CAD build for the part. Positions are in the model's coordinates, mm. A direction names the side the tool comes from. Coordinates: 2 decimals unless noted, no trailing zeros. Order: outer loops, then holes, each group sorted by start corner. A loop starts at its lowest first (then second) coordinate and runs counter-clockwise, first axis right, second up. Notation, with made-up numbers: (56.5, 69.25) - (77.5, 69.25) arc R32 cw to (77.5, 104.25) - close; hole circle Ø10 at (85, -22.75). An arc over 180 degrees is marked (long way). Use one line per item in the form item = value.
```python
from build123d import *

# Parameters (mm, degrees)
SKETCH_R           = 56.5
PAD_DEPTH          = 35
SKETCH001_R        = 55
POCKET_DEPTH       = 33
SKETCH002_R        = 6.9
PAD001_DEPTH       = 110
CHAMFER_SIZE       = 1
CHAMFER001_SIZE    = 1
SKETCH006_R        = 10
POCKET002_DEPTH    = 5
POLARPATTERN_COUNT = 6


with BuildPart() as part:
    # Sketch → Pad (new body)
    with BuildSketch(Plane.XY):
        Circle(SKETCH_R)
    extrude(amount=PAD_DEPTH)

    # Sketch001 (on Face3 of Pad) → Pocket (cut)
    with BuildSketch(Plane.XY.offset(35)):
        Circle(SKETCH001_R)
    extrude(amount=-POCKET_DEPTH, mode=Mode.SUBTRACT)

    # Sketch002 → Pad001 (join)
    with BuildSketch(Plane.XY):
        with Locations((0, -0.437585)):
            Circle(SKETCH002_R)
    extrude(amount=PAD001_DEPTH)

    # Chamfer
    chamfer_edges = [part.edges().sort_by_distance(p)[0] for p in [
        (-6.9, -0.437585, 110),
    ]]
    chamfer(chamfer_edges, length=CHAMFER_SIZE)

    # Chamfer001
    chamfer001_edges = [part.edges().sort_by_distance(p)[0] for p in [
        (-56.5, 0, 0),
    ]]
    chamfer(chamfer001_edges, length=CHAMFER001_SIZE)

    # Sketch006 (on Face6 of Pad001) → Pocket002 (cut)
    with BuildSketch(Plane.XY.offset(2)):
        with Locations((-25, 25)):
            Circle(SKETCH006_R)
    pocket002 = extrude(amount=-POCKET002_DEPTH, mode=Mode.SUBTRACT)

    # PolarPattern: Pocket002 ×6 about axis
    polarpattern_axis = Axis((0, 0, 2), (0, 0, 1))
    for i in range(1, POLARPATTERN_COUNT):
        add(pocket002.rotate(polarpattern_axis, i * 360 / POLARPATTERN_COUNT), mode=Mode.SUBTRACT)


solid = part.part
```
Item 1: Two-plate mould, pull along Y, no slides. Class faces 3 (the face through (12, -54, 35)), 4 (the face through (-1, -11, 2)), 5 (the face through (-11.923, -53.692, 18.731)), 6 (the face through (30.374, 47.641, 17.762)): +Y half, -Y half, draft (parallel to the pull), parting line (faces both ways), or undercut.
Derived:
face_3 = draft
face_4 = undercut
face_5 = undercut
face_6 = parting line
Item 2: Cut at A-A, the plane z = 28. Write the cut outline in (x, y), plus the area to 3 significant figures.
Derived:
outline = circle Ø113 at (0, 0); circle Ø13.8 at (0, -0.44); hole circle Ø110 at (0, 0)
area = 675 mm²
Item 3: Drill centre lines: line 1 (Y direction, x = 25, z = 1.15); line 2 (Z direction, x = -45, y = 26.5); line 3 (X direction, y = 46, z = 12). Where is each one in solid material? Low to high. Write a range as [from, to].
Derived:
line_1 = [-50.67, -35], [-15, 5.12], [13.18, 50.67]
line_2 = [0, 2]
line_3 = [-32.81, -30.15], [30.15, 32.81]
Item 4: Drop flat-ended pins along their axis: pin 1 (2 mm diameter, centred on x = 37, y = -31.5, fed in from +Z); pin 2 (6 mm diameter, centred on x = -9, z = 73.5, fed in from +Y). Give the stop position or say it passes through.
Derived:
pin_1 = 2
pin_2 = 2.97
Item 5: Cut at B-B, the plane z = 49.5. Write the cut outline in (x, y), plus the area to 3 significant figures.
Derived:
outline = circle Ø13.8 at (0, -0.44)
area = 150 mm²
Item 6: 3-axis set-ups, long thin cutter, end or side, ignore diameter. For faces 1 (the face through (-0.898, 6.404, 54.751)), 2 (the face through (24.16, 9.59, 1.01)): which of +Z, -Z, +X, -X, +Y, -Y reach the whole face in a straight line?
Derived:
face_1 = +Z
face_2 = +Z, -Z
